Check sheet for the drawn part. Datum: minimum x, y, z corner. Units: mm. A direction names the side the tool comes from. Coordinates: 2 decimals unless noted, no trailing zeros. Write each loop counter-clockwise with the first axis right and the second up, starting at its lowest first coordinate (ties: lowest second). Pieces come first, ordered by that corner, then holes. Notation, with made-up numbers: (52, -6) -> (61, -6) arc R30 ccw to (61, 28) -> close; hole circle Ø11 at (82, 31.5). An arc over 180 degrees is marked (long way). Answer in a Markdown table with one row per item.
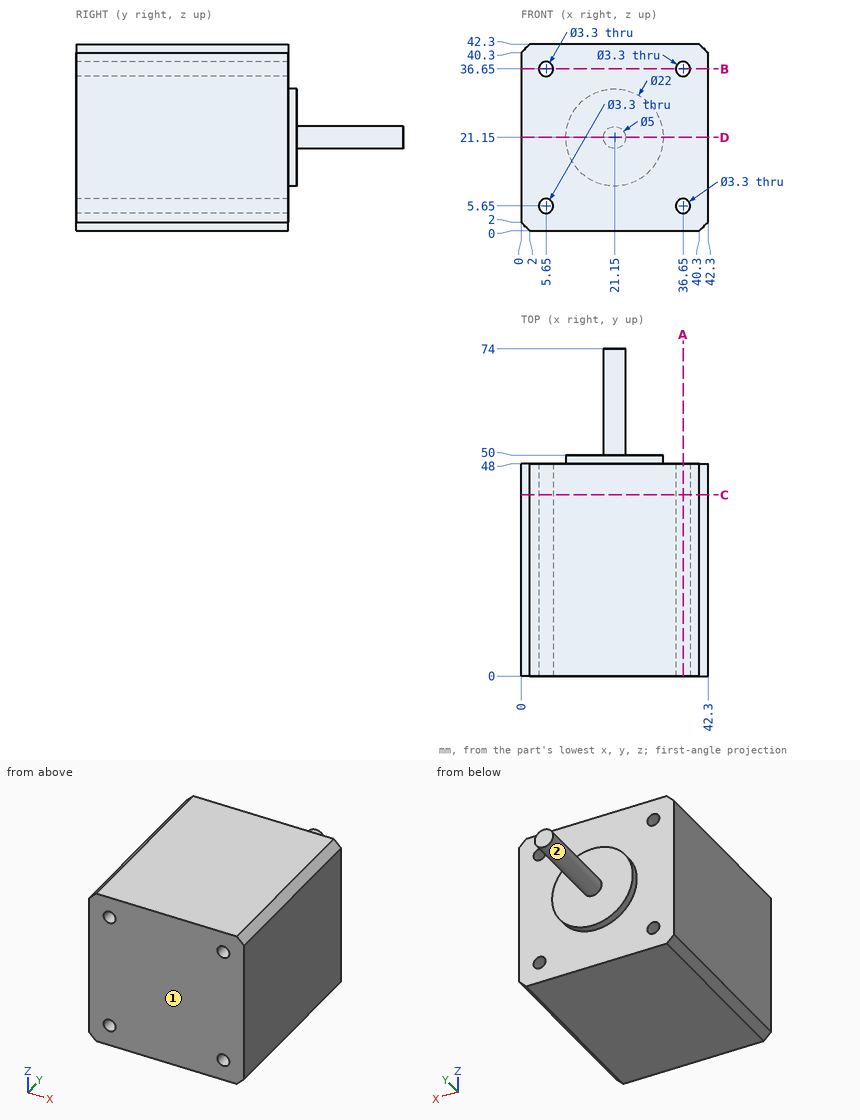
1. Sectioned sample at C-C, the plane y = 41. Record the cut outline in (x, z), and give its area (3 significant figures).
Findings below:
| item | result |
|---|---|
| outline | (0, 2) -> (2, 0) -> (40.3, 0) -> (42.3, 2) -> (42.3, 40.3) -> (40.3, 42.3) -> (2, 42.3) -> (0, 40.3) -> close; hole circle Ø3.3 at (5.65, 5.65); hole circle Ø3.3 at (5.65, 36.65); hole circle Ø3.3 at (36.65, 5.65); hole circle Ø3.3 at (36.65, 36.65) |
| area | 1,750 mm² |
2. Sectioned sample at D-D, the plane z = 21.15. Record the cut outline in (x, y).
Findings below:
| item | result |
|---|---|
| outline | (0, 0) -> (42.3, 0) -> (42.3, 48) -> (32.15, 48) -> (32.15, 50) -> (23.65, 50) -> (23.65, 74) -> (18.65, 74) -> (18.65, 50) -> (10.15, 50) -> (10.15, 48) -> (0, 48) -> close |
3. Sectioned sample at B-B, the plane z = 36.65. Record the cut outline in (x, y), and give its area (3 significant figures).
Findings below:
| item | result |
|---|---|
| outline | (0, 0) -> (4, 0) -> (4, 48) -> (0, 48) -> close; (7.3, 0) -> (35, 0) -> (35, 48) -> (7.3, 48) -> close; (38.3, 0) -> (42.3, 0) -> (42.3, 48) -> (38.3, 48) -> close |
| area | 1,710 mm² |
4. Sectioned sample at A-A, the plane x = 36.65. Record the cut outline in (y, z), and give its area (3 significant figures).
Findings below:
| item | result |
|---|---|
| outline | (0, 0) -> (48, 0) -> (48, 4) -> (0, 4) -> close; (0, 7.3) -> (48, 7.3) -> (48, 35) -> (0, 35) -> close; (0, 38.3) -> (48, 38.3) -> (48, 42.3) -> (0, 42.3) -> close |
| area | 1,710 mm² |
5. Go/stop test with flat-tipped pins: pin 1 (8 mm diameter, centred on x = 19, y = 58, fed in from -Z); pin 2 (2 mm diameter, centred on x = 5.65, z = 5.65, fed in from +Y); pin 3 (8 mm diameter, centred on x = 15, z = 5, fed in from +Y); pin 4 (21 mm diameter, centred on x = 31, z = 30, fed in from +Y). Record where each tip stops, or that it passes through.
Findings below:
| item | result |
|---|---|
| pin 1 | stops at z = 18.65 |
| pin 2 | passes through |
| pin 3 | stops at y = 48 |
| pin 4 | stops at y = 50 |
6. Material ranges on probe 1 along X at (y, z) = (18.5, 5.65); probe 2 along Z at (x, y) = (5, 31), recorded low to high. Write a range as from..to.
Findings below:
| item | result |
|---|---|
| probe 1 | x = 0..4, 7.3..35, 38.3..42.3 |
| probe 2 | z = 0..4.13, 7.17..35.13, 38.17..42.3 |
7. Access from +Z, -Z, +X, -X, +Y, -Y to the whole of each face (thin tool, end or side, straight path). Record for the marked faces 1 and 2.
Findings below:
| item | result |
|---|---|
| face 1 | +Z, -Z, +X, -X, -Y |
| face 2 | +Y |
